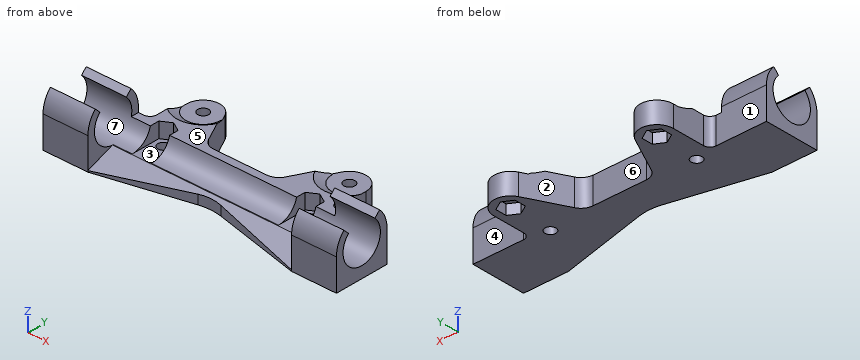
```python
from build123d import *

# Parameters (mm, degrees)
BOSS_EXTRUDE1_DEPTH = 88.3
SKETCH6_R           = 1.65
BOSS_EXTRUDE2_DEPTH = 8
CUT_EXTRUDE1_DEPTH  = 93.261259475
SKETCH8_W           = 61.3
SKETCH8_H           = 21.483950942
CUT_EXTRUDE2_DEPTH  = 93.118890571
SKETCH9_W           = 61.3
SKETCH9_H           = 11.699409457
CUT_EXTRUDE3_DEPTH  = 93.543511645
SKETCH10_R          = 1.65
CUT_EXTRUDE4_DEPTH  = 94.043055829
CHAMFER1_SIZE       = 8
CHAMFER1_SIZE2      = 3
CUT_EXTRUDE5_DEPTH  = 93.54351174
FILLET1_R           = 2
CUT_EXTRUDE6_DEPTH  = 3
CUT_EXTRUDE7_START  = -4.6
CUT_EXTRUDE7_DEPTH  = 4.6
CUT_EXTRUDE8_START  = -1.6
CUT_EXTRUDE8_DEPTH  = 1.6
CHAMFER2_SIZE       = 1.732050808
CHAMFER2_SIZE_2     = 3


with BuildPart() as part:
    # Sketch1 → Boss-Extrude1 (new body)
    with BuildSketch(Plane.ZY):
        with BuildLine():
            Line((-9.5, 8.25), (-9.5, -8.25))
            Line((-9.5, -8.25), (0, -8.25))
            ThreePointArc((0, -8.25), (8.25, 0), (0, 8.25))
            Line((0, 8.25), (-9.5, 8.25))
        make_face()
    extrude(amount=BOSS_EXTRUDE1_DEPTH)

    # Sketch6 → Boss-Extrude2 (add)
    with BuildSketch(Plane(origin=(0, 0, -9.5), x_dir=(-1, 0, 0), z_dir=(0, 0, -1))):
        with BuildLine():
            Line((17.15, -8.25), (17.15, 20))
            ThreePointArc((17.15, 20), (20.99096395, 24.863808737), (26.612654174, 22.254931867))
            Line((26.612654174, 22.254931867), (32.579554775, 10.446054507))
            ThreePointArc((32.579554775, 10.446054507), (34.053942202, 8.842964487), (36.149678114, 8.25))
            Line((36.149678114, 8.25), (52.150321886, 8.25))
            ThreePointArc((52.150321886, 8.25), (54.246057798, 8.842964487), (55.720445225, 10.446054507))
            Line((55.720445225, 10.446054507), (61.687345826, 22.254931867))
            ThreePointArc((61.687345826, 22.254931867), (67.30903605, 24.863808737), (71.15, 20))
            Line((71.15, 20), (71.15, -8.25))
            Line((71.15, -8.25), (17.15, -8.25))
        make_face()
        with Locations((22.15, 20)):
            Circle(SKETCH6_R, mode=Mode.SUBTRACT)
        with Locations(Location((66.15, 20, 0), (0, 0, 180))):
            Circle(SKETCH6_R, mode=Mode.SUBTRACT)
    extrude(amount=-BOSS_EXTRUDE2_DEPTH)

    # Sketch7 → Cut-Extrude1 (cut, through all)
    with BuildSketch(Plane.ZY.offset(88.3)):
        with BuildLine():
            Line((13.481907846, 13.481907846), (4.313351365, 4.313351365))
            ThreePointArc((4.313351365, 4.313351365), (-6.1, 0), (4.313351365, -4.313351365))
            Line((4.313351365, -4.313351365), (13.481907846, -13.481907846))
            Line((13.481907846, -13.481907846), (13.481907846, 13.481907846))
        make_face()
    extrude(amount=-CUT_EXTRUDE1_DEPTH, mode=Mode.SUBTRACT)

    # Sketch8 → Cut-Extrude2 (cut, through all)
    with BuildSketch(Plane.XY.offset(-1.5)):
        with Locations((-44.15, -2.491975471)):
            Rectangle(SKETCH8_W, SKETCH8_H)
    extrude(amount=CUT_EXTRUDE2_DEPTH, mode=Mode.SUBTRACT)

    # Sketch9 → Cut-Extrude3 (cut, through all)
    with BuildSketch(Plane(origin=(0, 0, -6.1), x_dir=(-1, 0, 0), z_dir=(0, 0, -1))):
        with Locations((44.15, -5.849704729)):
            Rectangle(SKETCH9_W, SKETCH9_H)
    extrude(amount=-CUT_EXTRUDE3_DEPTH, mode=Mode.SUBTRACT)

    # Sketch10 → Cut-Extrude4 (cut, through all)
    with BuildSketch(Plane(origin=(0, 0, -9.5), x_dir=(-1, 0, 0), z_dir=(0, 0, -1))):
        with Locations((22.15, 7)):
            Circle(SKETCH10_R)
        with Locations((66.15, 7)):
            Circle(SKETCH10_R)
    extrude(amount=-CUT_EXTRUDE4_DEPTH, mode=Mode.SUBTRACT)

    # Chamfer1
    chamfer1_edges = [part.edges().sort_by_distance(p)[0] for p in [
        (-44.15, -8.25, -6.1),
    ]]
    chamfer1_side = [part.faces().sort_by_distance(p)[0] for p in [
        (-44.15, -4.125, -6.1),
    ]]
    chamfer(chamfer1_edges, length=CHAMFER1_SIZE, length2=CHAMFER1_SIZE2, reference=chamfer1_side[0])

    # Sketch11 → Cut-Extrude5 (cut, through all)
    with BuildSketch(Plane(origin=(0, 0, -6.1), x_dir=(-1, 0, 0), z_dir=(0, 0, -1))):
        with BuildLine():
            Line((74.8, -8.25), (47.5958626, -1.828822614))
            ThreePointArc((47.5958626, -1.828822614), (44.15, -1.427659244), (40.7041374, -1.828822614))
            Line((40.7041374, -1.828822614), (13.5, -8.25))
            Line((13.5, -8.25), (13.5, -16.427659244))
            Line((13.5, -16.427659244), (74.8, -16.427659244))
            Line((74.8, -16.427659244), (74.8, -8.25))
        make_face()
    extrude(amount=CUT_EXTRUDE5_DEPTH, mode=Mode.SUBTRACT)

    # Fillet1
    fillet1_edges = [part.edges().sort_by_distance(p)[0] for p in [
        (-17.15, 8.25, -5.5),
        (-71.15, 8.25, -5.5),
    ]]
    fillet(fillet1_edges, radius=FILLET1_R)

    # Sketch12 → Cut-Extrude6 (cut)
    with BuildSketch(Plane(origin=(0, 0, -9.5), x_dir=(-1, 0, 0), z_dir=(0, 0, -1))):
        Polygon((22.15, 16.651368439), (25.05, 18.325684219), (25.05, 21.674315781), (22.15, 23.348631561), (19.25, 21.674315781), (19.25, 18.325684219), align=None)
        Polygon((66.15, 16.651368439), (69.05, 18.325684219), (69.05, 21.674315781), (66.15, 23.348631561), (63.25, 21.674315781), (63.25, 18.325684219), align=None)
    extrude(amount=-CUT_EXTRUDE6_DEPTH, mode=Mode.SUBTRACT)

    # Sketch13 → Cut-Extrude7 (cut)
    with BuildSketch(Plane.XY.offset(-1.5).offset(CUT_EXTRUDE7_START)):
        Polygon((-69.05, -2.12397244), (-63.25, -2.12397244), (-63.25, 8.674315781), (-66.15, 10.348631561), (-69.05, 8.674315781), align=None)
        Polygon((-25.05, -2.12397244), (-19.25, -2.12397244), (-19.25, 8.674315781), (-22.15, 10.348631561), (-25.05, 8.674315781), align=None)
    extrude(amount=CUT_EXTRUDE7_DEPTH, mode=Mode.SUBTRACT)

    # Sketch14 → Cut-Extrude8 (cut)
    with BuildSketch(Plane.XY.offset(-1.5).offset(CUT_EXTRUDE8_START)):
        with BuildLine():
            Line((-61.15, 20), (-27.15, 20))
            ThreePointArc((-27.15, 20), (-18.614466094, 16.464466094), (-22.15, 25))
            Line((-22.15, 25), (-66.15, 25))
            ThreePointArc((-66.15, 25), (-69.685533906, 16.464466094), (-61.15, 20))
        make_face()
    extrude(amount=CUT_EXTRUDE8_DEPTH, mode=Mode.SUBTRACT)

    # Chamfer2
    # the kernel refuses this chamfer: 3, 1.732050808 mm, written as the material it takes off along each edge
    with BuildSketch(Plane(origin=(-22.15, 20, -1.5), x_dir=(-0.016047871272964892, 0.9998712246222542, 0), z_dir=(0.9998712246222542, 0.016047871272964892, 0))) as chamfer2_piece_1_section:
        Polygon((5, -CHAMFER2_SIZE), (5 + CHAMFER2_SIZE_2, 0), (5, 0), align=None)
    chamfer2_piece_1 = revolve(axis=Axis((-22.15, 20, -1.5), (0, 0, 1)), revolution_arc=358.160970471, mode=Mode.PRIVATE)
    chamfer2_piece_1 = split(chamfer2_piece_1, bisect_by=Plane(origin=(-17.15, 16.005759066, -2.231169886), z_dir=(-1, 0, 0)), keep=Keep.TOP, mode=Mode.PRIVATE)
    chamfer2_piece_1 = split(chamfer2_piece_1, bisect_by=Plane(origin=(-27.459187994, 16.005759066, -3.1), z_dir=(0, 0, 1)), keep=Keep.TOP, mode=Mode.PRIVATE)
    add(chamfer2_piece_1, mode=Mode.SUBTRACT)
    with BuildSketch(Plane(origin=(-22.15, 20, -1.5), x_dir=(-0.016047871272964892, 0.9998712246222542, 0), z_dir=(0.9998712246222542, 0.016047871272964892, 0))) as chamfer2_piece_2_section:
        Polygon((5, -CHAMFER2_SIZE), (5 + CHAMFER2_SIZE_2, 0), (5, 0), align=None)
    chamfer2_piece_2 = revolve(axis=Axis((-22.15, 20, -1.5), (0, 0, 1)), revolution_arc=358.160970471, mode=Mode.PRIVATE)
    chamfer2_piece_2 = split(chamfer2_piece_2, bisect_by=Plane(origin=(-17.15, 20, -1.92443376), z_dir=(1, 0, 0)), keep=Keep.TOP, mode=Mode.PRIVATE)
    chamfer2_piece_2 = split(chamfer2_piece_2, bisect_by=Plane(origin=(-16.215864926, 20, -3.1), z_dir=(0, 0, 1)), keep=Keep.TOP, mode=Mode.PRIVATE)
    add(chamfer2_piece_2, mode=Mode.SUBTRACT)
    with BuildSketch(Plane(origin=(-66.15, 20, -1.5), x_dir=(-0.016047871272962772, 0.9998712246222542, 0), z_dir=(0.9998712246222542, 0.016047871272962772, 0))) as chamfer2_piece_3_section:
        Polygon((5, -CHAMFER2_SIZE), (5 + CHAMFER2_SIZE_2, 0), (5, 0), align=None)
    chamfer2_piece_3 = revolve(axis=Axis((-66.15, 20, -1.5), (0, 0, 1)), revolution_arc=358.160970471, mode=Mode.PRIVATE)
    chamfer2_piece_3 = split(chamfer2_piece_3, bisect_by=Plane(origin=(-70.144240933, 25.309187993, -3.1), z_dir=(0, 0, 1)), keep=Keep.TOP, mode=Mode.PRIVATE)
    chamfer2_piece_3 = split(chamfer2_piece_3, bisect_by=Plane(origin=(-71.15, 25.309187993, -2.231169885), z_dir=(1, 0, 0)), keep=Keep.TOP, mode=Mode.PRIVATE)
    add(chamfer2_piece_3, mode=Mode.SUBTRACT)
    with BuildSketch(Plane(origin=(-66.15, 20, -1.5), x_dir=(-0.016047871272962772, 0.9998712246222542, 0), z_dir=(0.9998712246222542, 0.016047871272962772, 0))) as chamfer2_piece_4_section:
        Polygon((5, -CHAMFER2_SIZE), (5 + CHAMFER2_SIZE_2, 0), (5, 0), align=None)
    chamfer2_piece_4 = revolve(axis=Axis((-66.15, 20, -1.5), (0, 0, 1)), revolution_arc=358.160970471, mode=Mode.PRIVATE)
    chamfer2_piece_4 = split(chamfer2_piece_4, bisect_by=Plane(origin=(-72.084135074, 20, -3.1), z_dir=(0, 0, 1)), keep=Keep.TOP, mode=Mode.PRIVATE)
    chamfer2_piece_4 = split(chamfer2_piece_4, bisect_by=Plane(origin=(-71.15, 20, -1.92443376), z_dir=(-1, 0, 0)), keep=Keep.TOP, mode=Mode.PRIVATE)
    add(chamfer2_piece_4, mode=Mode.SUBTRACT)


solid = part.part
```
Read the model definition and answer for the solid it produces. Units are mm, in the model's axes. Face numbers are marked on the shaded views. A direction names the side the tool comes from. Coordinates: 2 decimals unless noted, no trailing zeros. Write each loop counter-clockwise with the first axis right and the second up, starting at its lowest first coordinate (ties: lowest second). Pieces come first, ordered by that corner, then holes. Notation, with made-up numbers: (1, -12.75) -> (31, -12.75) arc R17 cw to (31, 3.25) -> close; hole circle Ø4 at (3.5, 65). An arc over 180 degrees is marked (long way). Write item = value, one per line.
(1) Section A-A on z = 1.5 is taken. Write down the section's boundary in (x, y), plus the area to 3 significant figures.
From the geometry:
outline = (-88.3, -8.11) -> (-74.8, -8.11) -> (-74.8, -5.91) -> (-88.3, -5.91) -> close; (-88.3, 5.91) -> (-74.8, 5.91) -> (-74.8, 8.11) -> (-88.3, 8.11) -> close; (-13.5, -8.11) -> (0, -8.11) -> (0, -5.91) -> (-13.5, -5.91) -> close; (-13.5, 5.91) -> (0, 5.91) -> (0, 8.11) -> (-13.5, 8.11) -> close
area = 119 mm2
(2) For a pull along Y with two mould halves and no side action, classify the marked faces 5, 6 and 7 as +Y half, -Y half, draft (parallel to the pull), parting line (faces both ways), or undercut.
From the geometry:
face_5 = draft
face_6 = +Y half
face_7 = undercut
(3) Section B-B on y = 7 is taken. Write down the section's boundary in (x, z), plus the area to 3 significant figures.
From the geometry:
outline = (-88.3, -9.5) -> (-67.8, -9.5) -> (-67.8, -6.1) -> (-69.05, -6.1) -> (-69.05, -1.5) -> (-74.8, -1.5) -> (-74.8, 4.37) -> (-88.3, 4.37) -> close; (-64.5, -9.5) -> (-23.8, -9.5) -> (-23.8, -6.1) -> (-25.05, -6.1) -> (-25.05, -1.5) -> (-63.25, -1.5) -> (-63.25, -6.1) -> (-64.5, -6.1) -> close; (-20.5, -9.5) -> (0, -9.5) -> (0, 4.37) -> (-13.5, 4.37) -> (-13.5, -1.5) -> (-19.25, -1.5) -> (-19.25, -6.1) -> (-20.5, -6.1) -> close
area = 789 mm2
(4) Section D-D on y = 2.5 is taken. Write down the section's boundary in (x, z).
From the geometry:
outline = (-88.3, -9.5) -> (0, -9.5) -> (0, -5.56) -> (-19.25, -5.56) -> (-19.25, -6.1) -> (-25.05, -6.1) -> (-25.05, -5.56) -> (-63.25, -5.56) -> (-63.25, -6.1) -> (-69.05, -6.1) -> (-69.05, -5.56) -> (-88.3, -5.56) -> close
(5) Given pin 1 Ø3 at (x, y) = (-23, 20) entering from -Z; pin 2 Ø7.5 at (x, z) = (-77, -6) entering from +Y; pin 3 Ø1.5 at (y, z) = (19.5, -8.5) entering from +X, each flat-ended and moving along its own axis, determine where each tip first touches the part or whether it passes through.
From the geometry:
pin_1 = -6.5
pin_2 = 8.25
pin_3 = -17.15
(6) Which of the six approach directions +Z, -Z, +X, -X, +Y, -Y give full straight-line access (tool end or side, diameter ignored) to the marked faces 1, 2, 3 and 4?
From the geometry:
face_1 = +Z, -Z, -X, +Y
face_2 = +Z, -Z, +Y
face_3 = +Z, -Y
face_4 = +Z, -Z, +X, +Y
(7) Section C-C on x = -33.5 is taken. Write down the section's boundary in (y, z).
From the geometry:
outline = (-3.53, -9.5) -> (9.25, -9.5) -> (9.25, -1.5) -> (5.91, -1.5) arc R6.1 cw to (0, -6.1) -> (-0.25, -6.1) -> (-3.53, -7.33) -> close
(8) Straight lines are drawn through the part: L1, parallel to X at y = -3.5, z = -5.5; L2, parallel to Y at x = -66.15, z = -3.75; L3, parallel to X at y = 17.5, z = -6.75. For each, find the intervals that lie inside material, in ascending order. Write a range as from..to.
From the geometry:
L1 = -88.3..-74.8, -13.5..0
L2 = 10.35..18.35, 21.65..25
L3 = -71.15..-67.62, -64.68..-59.28, -29.02..-23.62, -20.68..-17.15
